Verification items for the finished model (mm, model axes). Face numbers are marked on the shaded views. A direction names the side the tool comes from. Give positions to 0.01 mm unless a question says otherwise; leave off trailing zeros. Order: outer loops, then holes, each group sorted by start corner. A loop starts at its lowest first (then second) coordinate and runs counter-clockwise, first axis right, second up. Notation, with made-up numbers: (79, 36.5) -> (136, 36.5) arc R22 cw to (136, 44.5) -> close; hole circle Ø1 at (81.25, -4). An arc over 180 degrees is marked (long way). Write each question's results on one line, items separated by ' | '. Start each with the question number.
1. Cross-section at B-B, the plane x = 10.75. Enter the section's corners in (y, z), then the cut area to 3 significant figures.
2. Depth check by flat-ended pin: pin 1 Ø1.5 at (y, z) = (20, 0) entering from +X; pin 2 Ø7 at (x, z) = (-24.05, -4.95) entering from -Y; pin 3 Ø1.3 at (y, z) = (33, 1.5) entering from -X. Enter the tip coordinate at first touch or a pass-through.
3. Cross-section at C-C, the plane z = -0.25. Enter the section's corners in (x, y).
4. Material ranges on L1, parallel to X at y = 29.65, z = 4.95; L2, parallel to Z at x = -24.05, y = 29.8; L3, parallel to Y at x = 1.5, z = -5.75, recorded low to high. Write a range as from..to.
5. Cross-section at A-A, the plane z = -4.95. Enter the section's corners in (x, y), then the cut area to 3 significant figures.
6. Set-up check for the marked faces 1, 2 and 3: record each of +Z, -Z, +X, -X, +Y, -Y from which the full face is reachable in a straight line by a thin tool's end or side.
7. Cross-section at D-D, the plane y = 39. Enter the section's corners in (x, z).
from build123d import *

# Parameters (mm, degrees)
SKETCH1_W            = 39.5
SKETCH1_H            = 21
BOSS_EXTRUDE1_DEPTH  = 36
SKETCH2_R            = 4
BOSS_EXTRUDE2_DEPTH  = 11.5
SKETCH4_W            = 21
SKETCH4_H            = 2.5
BOSS_EXTRUDE4_DEPTH  = 7.5
SKETCH5_R            = 2.2
CUT_EXTRUDE1_DEPTH   = 7.5
FILLET1_R            = 3
FILLET1_OF_MIRROR1_R = 3
CHAMFER1_SIZE        = 0.5


with BuildPart() as part:
    # Sketch1 → Boss-Extrude1 (new body)
    with BuildSketch(Plane(origin=(0, 0, 0), x_dir=(1, 0, 0), z_dir=(0, 1, 0))):
        Rectangle(SKETCH1_W, SKETCH1_H)
    extrude(amount=BOSS_EXTRUDE1_DEPTH)

    # Sketch2 → Boss-Extrude2 (add)
    with BuildSketch(Plane(origin=(0, 36, 0), x_dir=(1, 0, 0), z_dir=(0, 1, 0))):
        with Locations(Location((10.75, 0, 0), (0, 0, 90))):
            Circle(SKETCH2_R)
    extrude(amount=BOSS_EXTRUDE2_DEPTH)

    # Sketch4 → Boss-Extrude4 (add)
    with BuildSketch(Plane(origin=(19.75, 0, 0), x_dir=(0, 0, -1), z_dir=(1, 0, 0))):
        with Locations((0, 29.75)):
            Rectangle(SKETCH4_W, SKETCH4_H)
    boss_extrude4 = extrude(amount=BOSS_EXTRUDE4_DEPTH)

    # Sketch5 → Cut-Extrude1 (cut)
    with BuildSketch(Plane(origin=(0, 31, 0), x_dir=(1, 0, 0), z_dir=(0, 1, 0))):
        with Locations(Location((24.05, 4.95, 0), (0, 0, 270))):
            Circle(SKETCH5_R)
        with Locations(Location((24.05, -4.95, 0), (0, 0, 270))):
            Circle(SKETCH5_R)
    cut_extrude1 = extrude(amount=-CUT_EXTRUDE1_DEPTH, mode=Mode.SUBTRACT)

    # Fillet1
    fillet1_edges = [part.edges().sort_by_distance(p)[0] for p in [
        (27.25, 29.75, 10.5),
        (27.25, 29.75, -10.5),
    ]]
    fillet(fillet1_edges, radius=FILLET1_R)

    # Mirror1: Boss-Extrude4, Cut-Extrude1 across plane
    add(boss_extrude4.mirror(Plane(origin=(0, 0, 0), x_dir=(0, 0, 1), z_dir=(1, 0, 0))))
    add(cut_extrude1.mirror(Plane(origin=(0, 0, 0), x_dir=(0, 0, 1), z_dir=(1, 0, 0))), mode=Mode.SUBTRACT)

    # Fillet1 of Mirror1
    fillet1_of_mirror1_edges = [part.edges().sort_by_distance(p)[0] for p in [
        (-27.25, 29.75, 10.5),
        (-27.25, 29.75, -10.5),
    ]]
    fillet(fillet1_of_mirror1_edges, radius=FILLET1_OF_MIRROR1_R)

    # Chamfer1
    chamfer1_edges = [part.edges().sort_by_distance(p)[0] for p in [
        (-19.75, 36, 0),
        (0, 36, 10.5),
        (19.75, 36, 0),
        (0, 36, -10.5),
    ]]
    chamfer(chamfer1_edges, length=CHAMFER1_SIZE)


solid = part.part
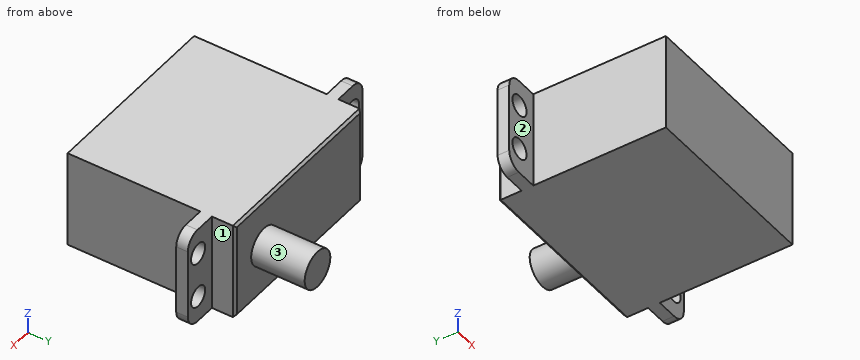
Results below:
1) outline: (0, -10.5) -> (35.5, -10.5) -> (36, -10) -> (36, -4) -> (47.5, -4) -> (47.5, 4) -> (36, 4) -> (36, 10) -> (35.5, 10.5) -> (0, 10.5) -> close | area: 848 mm²
2) pin 1: stops at x = 19.75 | pin 2: stops at y = 28.5 | pin 3: stops at x = -19.75
3) outline: (-27.25, 28.5) -> (-19.75, 28.5) -> (-19.75, 0) -> (19.75, 0) -> (19.75, 28.5) -> (27.25, 28.5) -> (27.25, 31) -> (19.75, 31) -> (19.75, 35.5) -> (19.25, 36) -> (14.74, 36) -> (14.74, 47.5) -> (6.76, 47.5) -> (6.76, 36) -> (-19.25, 36) -> (-19.75, 35.5) -> (-19.75, 31) -> (-27.25, 31) -> close
4) L1: x = -27.25..-26.25, -21.85..21.85, 26.25..27.25 | L2: z = -10.5..-7.15, -2.75..2.75, 7.15..10.5 | L3: y = 0..36
5) outline: (-27.25, 28.5) -> (-26.25, 28.5) -> (-26.25, 31) -> (-27.25, 31) -> close; (-21.85, 28.5) -> (-19.75, 28.5) -> (-19.75, 0) -> (19.75, 0) -> (19.75, 28.5) -> (21.85, 28.5) -> (21.85, 31) -> (19.75, 31) -> (19.75, 35.5) -> (19.25, 36) -> (-19.25, 36) -> (-19.75, 35.5) -> (-19.75, 31) -> (-21.85, 31) -> close; (26.25, 28.5) -> (27.25, 28.5) -> (27.25, 31) -> (26.25, 31) -> close | area: 1,440 mm²
6) face 1: +Z, -Z, +X, +Y | face 2: +Z, -Z, -X, -Y | face 3: +Y
7) outline: circle Ø8 at (10.75, 0)
